from build123d import *

# Parameters (mm, degrees)
F0_R     = 25.4
F1_DEPTH = 3.175
F2_R     = 25.4
F2_R_2   = 22.225
F3_DEPTH = 25.4
F4_D     = 5


with BuildPart() as f1:
    # F0 (on Top) → F1 (new body)
    with BuildSketch(Plane.XY):
        Circle(F0_R)
    extrude(amount=F1_DEPTH)

    # F2 (on face) → F3 (join)
    with BuildSketch(Plane.XY.offset(3.175)):
        Circle(F2_R)
        Circle(F2_R_2, mode=Mode.SUBTRACT)
    extrude(amount=F3_DEPTH)

    # F4 (through all)
    with Locations(Plane(origin=(0, 0, 0), x_dir=(1, 0, 0), z_dir=(0, 0, -1))):
        with Locations((0, 0)):
            Hole(F4_D / 2)


solid = f1.part
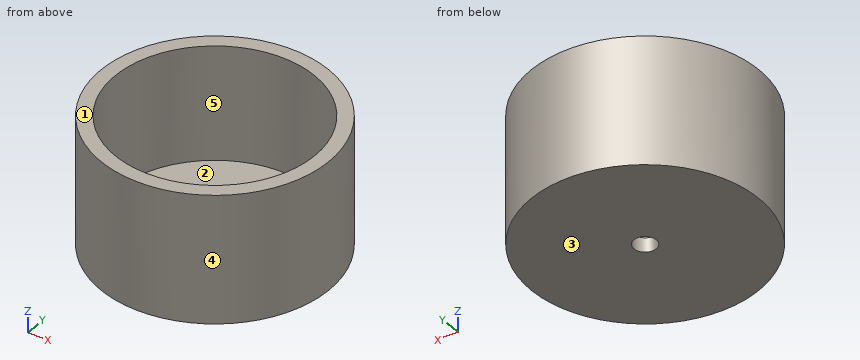
Input: part model. Units: mm. Frame: model coordinates. Face numbers are marked on the shaded views. A direction names the side the tool comes from. Give positions to 0.01 mm unless a question says otherwise; leave off trailing zeros. Order: outer loops, then holes, each group sorted by start corner. A loop starts at its lowest first (then second) coordinate and runs counter-clockwise, first axis right, second up. Notation, with made-up numbers: M 5.25,86.25 L 15.25,86.25 A15 ccw 15.25,92.25 Z; hole C -1.75,41.25 d11. An arc over 180 degrees is marked long. Answer as a JSON object with one key per item and string values.
1. Cut plane D-D, the plane y = 11. Output: boundary loops of the cut face in (x, z) (3 decimals).
Result sheet:
{"outline": "M -22.895,0 L 22.895,0 L 22.895,28.575 L 19.312,28.575 L 19.312,3.175 L -19.312,3.175 L -19.312,28.575 L -22.895,28.575 Z"}
2. First-contact query: P1, Ø5, axis at y = 10.5, z = 11, coming from the +X side; P2, Ø2, axis at y = 10, z = 21, coming from the +X side; P3, Ø22, axis at x = -9.5, y = -3.5, coming from the +Z side (3 decimals). Flat tips, straight axial feed; report the tip coordinate or a pass-through.
Result sheet:
{"P1": "x = 24.11", "P2": "x = 23.75", "P3": "z = 3.175"}
3. Cut plane B-B, the plane z = 25. Output: boundary loops of the cut face in (x, y) (3 decimals), and give its area (3 significant figures).
Result sheet:
{"outline": "C 0,0 d50.8; hole C 0,0 d44.45", "area": "475 mm²"}
4. Cut plane A-A, the plane x = 0. Output: boundary loops of the cut face in (y, z) (3 decimals), and give its area (3 significant figures).
Result sheet:
{"outline": "M -25.4,0 L -2.5,0 L -2.5,3.175 L -22.225,3.175 L -22.225,28.575 L -25.4,28.575 Z; M 2.5,0 L 25.4,0 L 25.4,28.575 L 22.225,28.575 L 22.225,3.175 L 2.5,3.175 Z", "area": "307 mm²"}
5. Ray query, line 1 (Y direction, x = 0, z = 1.3); line 2 (Y direction, x = 0, z = 12.5) (3 decimals); line 3 (Z direction, x = 7, y = -14) (3 decimals). Return the intervals inside material, ascending. Write a range as [from, to].
Result sheet:
{"line 1": "[-25.4, -2.5], [2.5, 25.4]", "line 2": "[-25.4, -22.225], [22.225, 25.4]", "line 3": "[0, 3.175]"}
6. Cut plane C-C, the plane y = -1. Output: boundary loops of the cut face in (x, z) (1 decimal), and give its area (3 significant figures).
Result sheet:
{"outline": "M -25.4,0 L -2.3,0 L -2.3,3.2 L -22.2,3.2 L -22.2,28.6 L -25.4,28.6 Z; M 2.3,0 L 25.4,0 L 25.4,28.6 L 22.2,28.6 L 22.2,3.2 L 2.3,3.2 Z", "area": "308 mm²"}
7. Reachability of the marked faces 1 and 2 from +Z, -Z, +X, -X, +Y, -Y: full face, straight path, thin tool, end or side. Return the list, or none.
Result sheet:
{"face 1": "+Z, +X, -X, +Y, -Y", "face 2": "+Z"}
8. Pull-direction query (Y, two-part tool) for the marked faces 3, 4 and 5; classes: +Y half, -Y half, draft (parallel to the pull), parting line (faces both ways), or undercut.
Result sheet:
{"face 3": "draft", "face 4": "parting line", "face 5": "undercut"}
